```python
from build123d import *

# Parameters (mm, degrees)
PAD_DEPTH       = 100
SKETCH001_R     = 5
POCKET_DEPTH    = 60.001
SKETCH002_W     = 24
SKETCH002_H     = 92
POCKET001_DEPTH = 110.001


with BuildPart() as part:
    # Sketch → Pad (new body)
    with BuildSketch(Plane.XY):
        with BuildLine():
            Line((100, 0), (100, 50))
            Line((100, 50), (0, 50))
            Line((0, 50), (0, 51))
            Line((0, 51), (90.050126, 51))
            ThreePointArc((102, 40.202041), (106.704409, 57.419629), (90.050126, 51))
            Line((102, 40.202041), (102, 0))
            Line((102, 0), (100, 0))
        make_face()
    extrude(amount=PAD_DEPTH)

    # Sketch001 → Pocket (cut, through all)
    with BuildSketch(Plane.XZ):
        with Locations((3.333333, 50)):
            Circle(SKETCH001_R)
        with Locations((51.666667, 50)):
            Circle(SKETCH001_R)
    extrude(amount=-POCKET_DEPTH, mode=Mode.SUBTRACT)

    # Sketch002 → Pocket001 (cut, through all)
    with BuildSketch(Plane.YZ):
        with Locations((12, 50)):
            Rectangle(SKETCH002_W, SKETCH002_H)
    extrude(amount=POCKET001_DEPTH, mode=Mode.SUBTRACT)


solid = part.part
```
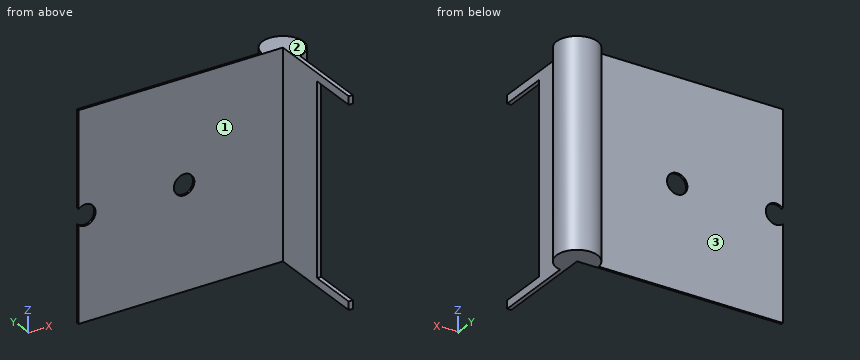
Build history of the part. All positions in model axes, mm. Face numbers are marked on the shaded views. A direction names the side the tool comes from. Round coordinates to 2 decimals unless told otherwise and drop trailing zeros. Loops run counter-clockwise (first coordinate to the right, second up) from the corner with the lowest first, then second, coordinate; pieces in that order, holes last. Notation, with made-up numbers: M -17,60.25 L 33,60.25 A15 cw 33,81.25 Z; hole C -2,8.5 d4. An arc over 180 degrees is marked long. Answer as CSV lines item,"result".
1. Wall check: probe 1 along Y at (x, z) = (38, 91.5); probe 2 along X at (y, z) = (31, 82); probe 3 along Y at (x, z) = (102.5, 41.5). Give the ranges that are in metal, low to high. Write a range as [from, to].
Resolved:
probe 1,"y = [50, 51]"
probe 2,"x = [100, 102]"
probe 3,"y = [40.32, 59.68]"
2. Cut at B-B on x = 55. Write the cut outline in (y, z), then the cut area to 3 significant figures.
Resolved:
outline,"M 50,0 L 51,0 L 51,46.27 L 50,46.27 Z; M 50,53.73 L 51,53.73 L 51,100 L 50,100 Z"
area,"92.5 mm²"
3. 3-axis set-ups, long thin cutter, end or side, ignore diameter. For the marked faces 1, 2 and 3: which of +Z, -Z, +X, -X, +Y, -Y reach the whole face in a straight line?
Resolved:
face 1,"+Z, -Z, -X, -Y"
face 2,"+Z, +X, -X, +Y, -Y"
face 3,"+Z, -Z, -X, +Y"
4. Flat gauge pins, fed straight in: P1, Ø1.5, axis at y = 40.5, z = 46.5, coming from the -X side; P2, Ø12, axis at y = 14.5, z = 60, coming from the +X side; P3, Ø6, axis at x = 14.5, z = 33, coming from the -Y side; P4, Ø2, axis at x = 101.5, z = 37, coming from the -Y side. Where does each tip first touch, or does it go through?
Resolved:
P1,"stops at x = 100"
P2,"passes through"
P3,"stops at y = 50"
P4,"stops at y = 24"
5. Cut at D-D on x = 10.5. Write the cut outline in (y, z).
Resolved:
outline,"M 50,0 L 51,0 L 51,100 L 50,100 Z"
6. Cut at A-A on z = 50. Write the cut outline in (x, y), then the cut area to 3 significant figures.
Resolved:
outline,"M 8.33,50 L 46.67,50 L 46.67,51 L 8.33,51 Z; M 56.67,50 L 100,50 L 100,24 L 102,24 L 102,40.2 A10 ccw long 90.05,51 L 56.67,51 Z"
area,"339 mm²"
7. Cut at C-C on z = 30. Write the cut outline in (x, y).
Resolved:
outline,"M 0,50 L 100,50 L 100,24 L 102,24 L 102,40.2 A10 ccw long 90.05,51 L 0,51 Z"
